Could you check a few things on this model? Use its own coordinates, in mm. Face numbers are marked on the shaded views. A direction names the side the tool comes from. Give positions to 0.01 mm unless a question says otherwise; leave off trailing zeros. Write each loop counter-clockwise with the first axis right and the second up, starting at its lowest first coordinate (ties: lowest second). Pieces come first, ordered by that corner, then holes. Notation, with made-up numbers: M -7,23.25 L 18,23.25 A19 cw 18,35.25 Z; hole C 10,79.25 d11. An arc over 180 degrees is marked long. Use one line per item in the form item = value.
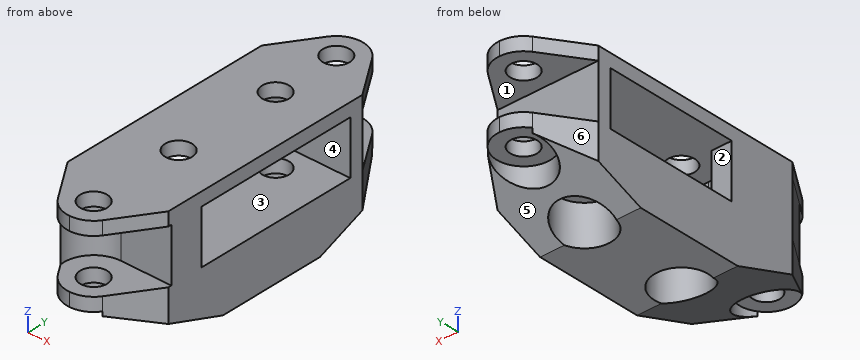
from build123d import *

# Parameters (mm, degrees)
SKETCH1_W               = 23.8125
SKETCH1_H               = 76.2
BOSS_EXTRUDE1_DEPTH     = 28.575
SKETCH2_R               = 3.175
CUT_EXTRUDE1_DEPTH      = 31.75
SKETCH11_W              = 12.7
SKETCH11_H              = 12.7
SKETCH11_H_2            = 60.325
CUT_EXTRUDE7_DEPTH      = 12.90625
CUT_EXTRUDE7_DEPTH_BACK = 12.90625
BOSS_EXTRUDE3_DEPTH     = 12.7
CUT_EXTRUDE8_START      = -3.175
SKETCH13_R              = 6.35
CUT_EXTRUDE8_DEPTH      = 10.525


with BuildPart() as part:
    # Sketch1 → Boss-Extrude1 (new body)
    with BuildSketch(Plane.XY):
        Rectangle(SKETCH1_W, SKETCH1_H)
    extrude(amount=BOSS_EXTRUDE1_DEPTH)

    # Sketch2 → Cut-Extrude1 (cut)
    with BuildSketch(Plane.XY.offset(28.575)):
        with BuildLine():
            Line((-11.90625, -38.1), (0, -38.1))
            ThreePointArc((0, -38.1), (-2.988235294, -37.352941176), (-5.273356401, -35.287543253))
            Line((-5.273356401, -35.287543253), (-11.90625, -25.4))
            Line((-11.90625, -25.4), (-11.90625, -38.1))
        make_face()
        with BuildLine():
            Line((11.90625, -38.1), (11.90625, -25.4))
            Line((11.90625, -25.4), (5.273356401, -35.287543253))
            ThreePointArc((5.273356401, -35.287543253), (2.988235294, -37.352941176), (0, -38.1))
            Line((0, -38.1), (11.90625, -38.1))
        make_face()
        with BuildLine():
            ThreePointArc((0, 38.1), (2.988235294, 37.352941176), (5.273356401, 35.287543253))
            Line((5.273356401, 35.287543253), (11.90625, 25.4))
            Line((11.90625, 25.4), (11.90625, 38.1))
            Line((11.90625, 38.1), (0, 38.1))
        make_face()
        with BuildLine():
            ThreePointArc((-5.273356401, 35.287543253), (-2.988235294, 37.352941176), (0, 38.1))
            Line((0, 38.1), (-11.90625, 38.1))
            Line((-11.90625, 38.1), (-11.90625, 25.4))
            Line((-11.90625, 25.4), (-5.273356401, 35.287543253))
        make_face()
        with Locations((0, 31.75)):
            Circle(SKETCH2_R)
        with Locations((0, 15.875)):
            Circle(SKETCH2_R)
        with Locations((0, -9.525)):
            Circle(SKETCH2_R)
        with Locations((0, -31.75)):
            Circle(SKETCH2_R)
    extrude(amount=-CUT_EXTRUDE1_DEPTH, mode=Mode.SUBTRACT)

    # Sketch11 → Cut-Extrude7 (cut, two sides)
    with BuildSketch(Plane(origin=(0, 0, 0), x_dir=(0, 0, -1), z_dir=(1, 0, 0))) as cut_extrude7_sk:
        with Locations((-19.05, 31.75)):
            Rectangle(SKETCH11_W, SKETCH11_H)
        with Locations((-19.05, -7.9375)):
            Rectangle(SKETCH11_W, SKETCH11_H_2)
        Polygon((0, 14.2875), (-9.525, 38.1), (0, 38.1), align=None)
        Polygon((0, -11.1125), (-9.525, -38.1), (0, -38.1), align=None)
    extrude(amount=CUT_EXTRUDE7_DEPTH, mode=Mode.SUBTRACT)
    extrude(cut_extrude7_sk.sketch, amount=-CUT_EXTRUDE7_DEPTH_BACK, mode=Mode.SUBTRACT)

    # Sketch12 → Boss-Extrude3 (add)
    with BuildSketch(Plane(origin=(0, 0, 25.4), x_dir=(-1, 0, 0), z_dir=(0, 0, -1))):
        with BuildLine():
            Line((0, -24.60625), (-11.90625, -24.60625))
            Line((-11.90625, -24.60625), (-11.90625, -16.66875))
            Line((-11.90625, -16.66875), (0, -16.66875))
            ThreePointArc((0, -16.66875), (5.051394068, -14.576394068), (7.14375, -9.525))
            Line((7.14375, -9.525), (11.90625, -9.525))
            Line((11.90625, -9.525), (11.90625, -25.4))
            Line((11.90625, -25.4), (7.096564462, -32.569717572))
            ThreePointArc((7.096564462, -32.569717572), (5.333339548, -26.997247815), (0, -24.60625))
        make_face()
    extrude(amount=BOSS_EXTRUDE3_DEPTH)

    # Sketch13 → Cut-Extrude8 (cut, through all)
    with BuildSketch(Plane.XY.offset(12.7).offset(CUT_EXTRUDE8_START)):
        with Locations((0, 31.75)):
            Circle(SKETCH13_R)
        with Locations((0, 15.875)):
            Circle(SKETCH13_R)
        with Locations((0, -9.525)):
            Circle(SKETCH13_R)
        with Locations((0, -31.75)):
            Circle(SKETCH13_R)
    extrude(amount=-CUT_EXTRUDE8_DEPTH, mode=Mode.SUBTRACT)


solid = part.part
1) For the marked faces 1, 2 and 3, which set-ups out of +Z, -Z, +X, -X, +Y, -Y let a thin tool reach every point of the face, with its end or its side?
Checked values:
face_1 = +X, -X, +Y
face_2 = +X, -X
face_3 = +X
2) For pin 1 Ø6.5 at (x, z) = (-2.5, 21.5) entering from -Y; pin 2 Ø11.5 at (x, y) = (0, 31.75) entering from +Z (3 decimals); pin 3 Ø4 at (x, z) = (-10.5, 18) entering from +Y; pin 4 Ø2 at (y, z) = (6.5, 14.5) entering from -X, each with a flat end and sliding along its axis, tell me the tip position at first contact or that it passes through.
Checked values:
pin_1 = -27.51
pin_2 = 28.575
pin_3 = 25.4
pin_4 = through
3) I want a section at A-A, the plane y = -31.75. Please give me the cut outline in (x, z) (3 decimals), plus the area to 3 significant figures.
Checked values:
outline = M -7.646,7.284 L -6.35,7.284 L -6.35,9.525 L -3.175,9.525 L -3.175,12.7 L -7.144,12.7 L -7.144,25.4 L -3.175,25.4 L -3.175,28.575 L -7.646,28.575 Z; M 3.175,9.525 L 6.35,9.525 L 6.35,7.284 L 7.646,7.284 L 7.646,12.7 L 3.175,12.7 Z; M 3.175,25.4 L 7.646,25.4 L 7.646,28.575 L 3.175,28.575 Z
area = 69.0 mm2
4) If I drill on L1, parallel to Y at x = 0, z = 26.65 (3 decimals); L2, parallel to Z at x = -3.75, y = 32 (3 decimals); L3, parallel to Z at x = 10, y = -10 (3 decimals), over which ranges is the centre line in solid material (lowest first)?
Checked values:
L1 = -38.1 to -34.925, -28.575 to -12.7, -6.35 to 12.7, 19.05 to 28.575, 34.925 to 38.1
L2 = 9.525 to 12.7, 25.4 to 28.575
L3 = 0 to 12.7, 25.4 to 28.575
5) Thinking about a two-plate mould opening in Z: for the marked faces 4, 5 and 6, which applies, released by +Z, released by -Z, zero draft, split by the parting line, or undercut?
Checked values:
face_4 = undercut
face_5 = released by -Z
face_6 = zero draft
6) I want a section at C-C, the plane x = -8.25. Please give me the cut outline in (y, z) (1 decimal), plus the area to 3 significant figures.
Checked values:
outline = M -30.9,7 L -11.1,0 L 14.3,0 L 30.9,6.6 L 30.9,12.7 L 25.4,12.7 L 25.4,25.4 L 30.9,25.4 L 30.9,28.6 L -30.9,28.6 Z; hole M -9.5,12.7 L 22.2,12.7 L 22.2,25.4 L -9.5,25.4 Z
area = 1,170 mm2
